```python
from build123d import *

# Parameters (mm, degrees)
BOSS_EXTRUDE1_DEPTH = 10
SKETCH2_R           = 1.5
CUT_EXTRUDE1_DEPTH  = 10
SKETCH3_W           = 10
SKETCH3_H           = 15
BOSS_EXTRUDE2_DEPTH = 10
FILLET1_R           = 2
FILLET2_R           = 2


with BuildPart() as part:
    # Sketch1 → Boss-Extrude1 (new body)
    with BuildSketch(Plane.XY):
        with BuildLine():
            Line((75, 0), (0, 0))
            add(Edge.make_bspline(
                [(0, 0), (-35.458503055, -15.603734429), (-43, -53)],
                knots=[0, 0, 0, 1, 1, 1], degree=2))
            Line((-43, -53), (-40, -53))
            add(Edge.make_bspline(
                [(-40, -53), (-36.902106975, -38.240903448), (-29.221449222, -27)],
                knots=[0, 0, 0, 0.424675214, 0.424675214, 0.424675214], degree=2))
            Line((-29.221449222, -27), (104.220036535, -27))
            add(Edge.make_bspline(
                [(104.220036535, -27), (111.901041982, -38.240979318), (115, -53)],
                knots=[1.077789281, 1.077789281, 1.077789281, 1.502471236, 1.502471236, 1.502471236], degree=2))
            Line((115, -53), (118, -53))
            add(Edge.make_bspline(
                [(118, -53), (110.458503055, -15.603734429), (75, 0)],
                knots=[0.536217864, 0.536217864, 0.536217864, 1.536217864, 1.536217864, 1.536217864], degree=2))
        make_face()
        with BuildLine():
            add(Edge.make_bspline(
                [(-26.253921627, -23), (-16.272049525, -10.585512223), (0, -3)],
                knots=[0.502463919, 0.502463919, 0.502463919, 1, 1, 1], degree=2))
            Line((0, -3), (75, -3))
            add(Edge.make_bspline(
                [(75, -3), (91.270620149, -10.585764027), (101.252432073, -23)],
                knots=[0.502471236, 0.502471236, 0.502471236, 1, 1, 1], degree=2))
            Line((101.252432073, -23), (-26.253921627, -23))
        make_face(mode=Mode.SUBTRACT)
    extrude(amount=BOSS_EXTRUDE1_DEPTH)

    # Sketch2 → Cut-Extrude1 (cut)
    with BuildSketch(Plane(origin=(0, 0, 0), x_dir=(1, 0, 0), z_dir=(0, 1, 0))):
        with Locations((71.5, -5)):
            Circle(SKETCH2_R)
        with Locations((3.5, -5)):
            Circle(SKETCH2_R)
        with Locations((37.5, -5)):
            Circle(SKETCH2_R)
    extrude(amount=-CUT_EXTRUDE1_DEPTH, mode=Mode.SUBTRACT)

    # Sketch3 → Boss-Extrude2 (add)
    with BuildSketch(Plane.XZ.offset(53)):
        with Locations((116.5, 5)):
            Rectangle(SKETCH3_W, SKETCH3_H)
        with Locations((-41.5, 5)):
            Rectangle(SKETCH3_W, SKETCH3_H)
    extrude(amount=BOSS_EXTRUDE2_DEPTH)

    # Fillet1
    fillet1_edges = [part.edges().sort_by_distance(p)[0] for p in [
        (111.5, -58, 12.5),
        (111.5, -58, -2.5),
        (121.5, -58, -2.5),
        (121.5, -58, 12.5),
        (111.5, -63, 5),
        (116.5, -63, -2.5),
        (121.5, -63, 5),
        (116.5, -63, 12.5),
    ]]
    fillet(fillet1_edges, radius=FILLET1_R)

    # Fillet2
    fillet2_edges = [part.edges().sort_by_distance(p)[0] for p in [
        (-36.5, -58, 12.5),
        (-46.5, -58, 12.5),
        (-46.5, -58, -2.5),
        (-36.5, -58, -2.5),
        (-41.5, -63, 12.5),
        (-46.5, -63, 5),
        (-41.5, -63, -2.5),
        (-36.5, -63, 5),
    ]]
    fillet(fillet2_edges, radius=FILLET2_R)


solid = part.part
```
Geometry: final body of the model. Coordinates: model frame, mm. A direction names the side the tool comes from. Coordinates: 2 decimals unless noted, no trailing zeros. Write each loop counter-clockwise with the first axis right and the second up, starting at its lowest first coordinate (ties: lowest second). Pieces come first, ordered by that corner, then holes. Notation, with made-up numbers: M -18,58.5 L 16,58.5 A8 cw 16,73.5 Z; hole C 40,18 d5. An arc over 180 degrees is marked long. Use CSV: the item, a comma, the result in double quotes. Start each with the question number.
1. Reachability of faces 1 (the face through (36.3, -1.5, 5.9)), 2 (the face through (111.5, -57, 5)), 3 (the face through (-42, -57, 12.5)), 4 (the face through (37, -3, 3)) from +Z, -Z, +X, -X, +Y, -Y: full face, straight path, thin tool, end or side. Return the list, or none.
2. Cut plane C-C on z = 5. Count the separate pieces of the cut face and the enclosed holes in it, plus the area to 3 significant figures.
3. Mould query, pull axis Z, two halves, no side actions, for faces 5 (the face through (73, -1, 5)), 6 (the face through (116, -57, -2.5)), 7 (the face through (-46.5, -57, 5)). Classes: pulls with the +Z half, pulls with the -Z half, needs draft (parallel to the pull), parting line crosses it, or undercut.
4. Ray query, probe 1 along Y at (x, z) = (62, 0.25); probe 2 along X at (y, z) = (-55, 1.5); probe 3 along Z at (x, y) = (71.5, -0.8). Return the intervals inside material, ascending.
5. First-contact query: P1, Ø3, axis at x = 12, z = 4, coming from the -Y side; P2, Ø2, axis at x = 87.5, y = -24, coming from the -Z side; P3, Ø1.5, axis at y = -33, z = 7, coming from the -X side. Flat tips, straight axial feed; report the tip coordinate or a pass-through.
6. Cut plane B-B on x = 37.5. Return the cut outline in (y, z).
7. Cut plane A-A on x = 61. Return the cut outline in (y, z).
Entries:
1,face 1,"+Y"
1,face 2,"+Z, -Z, -Y"
1,face 3,"+Z, +X, -X, +Y, -Y"
1,face 4,"+Z, -Z"
2,separate pieces,"3"
2,enclosed holes,"0"
2,area,"1,320 mm²"
3,face 5,"undercut"
3,face 6,"pulls with the -Z half"
3,face 7,"needs draft"
4,probe 1,"-27 to -23, -3 to 0"
4,probe 2,"-46.5 to -36.5, 111.5 to 121.5"
4,probe 3,"0 to 3.5, 6.5 to 10"
5,P1,"y = -27"
5,P2,"z = 0"
5,P3,"x = -36.58"
6,outline,"M -27,0 L -23,0 L -23,10 L -27,10 Z; M -3,0 L 0,0 L 0,3.5 L -3,3.5 Z; M -3,6.5 L 0,6.5 L 0,10 L -3,10 Z"
7,outline,"M -27,0 L -23,0 L -23,10 L -27,10 Z; M -3,0 L 0,0 L 0,10 L -3,10 Z"
